Can you work these out from the model? Positions are in its coordinate system, mm. A direction names the side the tool comes from. Round coordinates to 2 decimals unless told otherwise and drop trailing zeros. Order: outer loops, then holes, each group sorted by start corner. A loop starts at its lowest first (then second) coordinate and runs counter-clockwise, first axis right, second up. Notation, with made-up numbers: (-11, -7) -> (38, -7) arc R23 cw to (38, 22) -> close; hole circle Ø9 at (9.25, 83). An arc over 180 degrees is marked (long way). Use a Markdown table: item, result. Add a question column.
Q1. We'd pull the mould along Y, two halves only. Please class faces 1 (the face through (1.464, 6.594, 47.156)), 2 (the face through (-10.073, -3.172, 25.261)), 3 (the face through (-0.1, 4.4, 53.55)): +Y half, -Y half, draft (parallel to the pull), parting line (faces both ways), or undercut.
Q2. For faces 4 (the face through (0, 0, 0)), 5 (the face through (-4.02, -1.27, 47.16)), 6 (the face through (0, 0, 2.54)), which set-ups out of +Z, -Z, +X, -X, +Y, -Y let a thin tool reach every point of the face, with its end or its side?
Q3. I'm going to push flat-ended pins straight in: pin 1 Ø5 at (x, y) = (2, 13) entering from +Z; pin 2 Ø4 at (x, y) = (-5.5, 14.5) entering from +Z; pin 3 Ø6 at (x, y) = (-13, -12.5) entering from +Z. Where does each tip first touch, or does it pass through?
Q4. If we section it at B-B on z = 12: List the corners of the cut face in (x, y) for me.
Q5. I need wall thicknesses on line 1 along X through (y, z) = (0, 50.75); line 2 along Z through (x, y) = (-5.5, -11.5). Which ranges of each line are inside material? Lowest first, please. Write a range as [from, to].
Q6. If we section it at A-A on z = 45: List the corners of the cut face in (x, y) for me.
```python
from build123d import *

# Parameters (mm, degrees)
F2_R = 5.08
F3_T = -2.54


with BuildPart() as f1:
    # F0 (on Front) → F1 (revolve)
    with BuildSketch(Plane.XZ):
        Polygon((-6.754948, 39.844375), (-24.768133, 0), (0, 0), (0, 53.550061), (-6.754948, 53.550061), align=None)
    revolve(axis=Axis((0, 0, 26.77503), (0, 0, 1)))

    # F2
    f2_edges = [f1.edges().sort_by_distance(p)[0] for p in [
        (6.754948, 0, 39.844375),
        (24.768133, 0, 0),
        (-15.76154, 0, 19.922188),
    ]]
    fillet(f2_edges, radius=F2_R)

    # F3
    f3_openings = [f1.faces().sort_by_distance(p)[0] for p in [
        (0, 0, 53.550061),
    ]]
    offset(amount=F3_T, openings=f3_openings)


solid = f1.part
```
Answer below:
| question | item | result |
|---|---|---|
| 1 | face 1 | parting line |
| 1 | face 2 | undercut |
| 1 | face 3 | draft |
| 2 | face 4 | -Z, +X, -X, +Y, -Y |
| 2 | face 5 | +Z |
| 2 | face 6 | none |
| 3 | pin 1 | z = 31.22 |
| 3 | pin 2 | z = 24.91 |
| 3 | pin 3 | z = 21.53 |
| 4 | outline | circle Ø38.69 at (0, 0); hole circle Ø33.11 at (0, 0) |
| 5 | line 1 | [-6.75, -4.21], [4.21, 6.75] |
| 5 | line 2 | [0, 2.54], [20.42, 26.59] |
| 6 | outline | circle Ø13.51 at (0, 0); hole circle Ø8.43 at (0, 0) |
